Geometry: final body of the model. Coordinates: model frame, mm. A direction names the side the tool comes from. Round coordinates to 2 decimals unless told otherwise and drop trailing zeros. Loops run counter-clockwise (first coordinate to the right, second up) from the corner with the lowest first, then second, coordinate; pieces in that order, holes last. Notation, with made-up numbers: (71, 79) - (105, 79) arc R32 ccw to (105, 112) - close; hole circle Ø5 at (-3, 21.5). An arc over 180 degrees is marked (long way). Use CSV: the item, a comma, the result in double quotes.
from build123d import *

# Parameters (mm, degrees)
F1_DEPTH  = 1.5875
F3_DEPTH  = 4.7625
F4_W      = 6.35
F4_H      = 6.35
F5_DEPTH  = 3.175
F6_SIZE   = 1.8598642
F7_W      = 28.575
F7_H      = 3.175
F8_DEPTH  = 1.5875
F9_W      = 25.4
F9_H      = 1.5875
F10_DEPTH = 7.9375
F11_R     = 1.0922
F11_R_2   = 1.63322
F12_DEPTH = 28.575
F13_SIZE  = 1.58749
F14_R     = 0.396875
F15_DEPTH = 7.9375
F16_R     = 1.63322
F17_DEPTH = 1.5875


# Not quite as in the source:
# - a fillet or chamfer is up to 0.001 mm smaller than in the source, because OpenCascade refuses the exact size


with BuildPart() as f1:
    # F0 (on Top) → F1 (new body)
    with BuildSketch(Plane.XY):
        Polygon((-87.87765, 25.4), (-127, 25.4), (-127, 20.6375), (-48.7553, 20.6375), (-23.3553, -4.7625), (23.3553, -4.7625), (48.7553, 20.6375), (127, 20.6375), (127, 25.4), (87.87765, 25.4), (46.7826079092, 49.1262336135), (-46.7826079092, 49.1262336135), align=None)
        Polygon((-21.3826079092, 0), (-46.7826079092, 25.4), (-78.35265, 25.4), (-45.5064998802, 44.3637336135), (45.5064998802, 44.3637336135), (78.35265, 25.4), (46.7826079092, 25.4), (21.3826079092, 0), align=None, mode=Mode.SUBTRACT)
    extrude(amount=F1_DEPTH)

    # F2 (on face) → F3 (join)
    with BuildSketch(Plane.XY.offset(1.5875)):
        Polygon((-127, 22.225), (-127, 20.6375), (-48.7553, 20.6375), (-23.3553, -4.7625), (23.3553, -4.7625), (48.7553, 20.6375), (127, 20.6375), (127, 22.225), (93.376911314, 22.225), (87.87765, 25.4), (46.7826079092, 49.1262336135), (-46.7826079092, 49.1262336135), (-87.87765, 25.4), (-93.376911314, 22.225), align=None)
        Polygon((90.201911314, 22.225), (48.0977359697, 22.225), (22.6977359697, -3.175), (14.2875, -3.175), (14.2875, -1.5875), (-14.2875, -1.5875), (-14.2875, -3.175), (-22.6977359697, -3.175), (-48.0977359697, 22.225), (-90.201911314, 22.225), (-46.3572385662, 47.5387336135), (-14.2875, 47.5387336135), (-14.2875, 45.9512336135), (14.2875, 45.9512336135), (14.2875, 47.5387336135), (46.3572385662, 47.5387336135), align=None, mode=Mode.SUBTRACT)
    extrude(amount=F3_DEPTH)

    # F4 (on face) → F5 (join, through all)
    with BuildSketch(Plane(origin=(0, 22.225, 0), x_dir=(-1, 0, 0), z_dir=(0, 1, 0))):
        with Locations((-53.5178, 3.175)):
            Rectangle(F4_W, F4_H)
        with Locations((-123.825, 3.175)):
            Rectangle(F4_W, F4_H)
        with Locations((123.825, 3.175)):
            Rectangle(F4_W, F4_H)
        with Locations((53.5178, 3.175)):
            Rectangle(F4_W, F4_H)
    extrude(amount=F5_DEPTH)

    # F6
    f6_edges = [f1.edges().sort_by_distance(p)[0] for p in [
        (-127, 23.01875, 6.35),
        (-120.65, 23.8125, 6.35),
        (-56.6928, 23.8125, 6.35),
        (-50.3428, 23.8125, 6.35),
        (50.3428, 23.8125, 6.35),
        (56.6928, 23.8125, 6.35),
        (120.65, 23.8125, 6.35),
        (127, 23.01875, 6.35),
    ]]
    chamfer(f6_edges, length=F6_SIZE)

    # F7 (on face) → F8 (join)
    with BuildSketch(Plane.XY.offset(6.35)):
        with Locations((0, -3.175)):
            Rectangle(F7_W, F7_H)
        with Locations((0, 47.5387336135)):
            Rectangle(F7_W, F7_H)
    extrude(amount=F8_DEPTH)

    # F9 (on face) → F10 (cut, through all)
    with BuildSketch(Plane.XY.offset(7.9375)):
        with Locations((0, -3.96875)):
            Rectangle(F9_W, F9_H)
        with Locations((0, 48.3324836135)):
            Rectangle(F9_W, F9_H)
    extrude(amount=-F10_DEPTH, mode=Mode.SUBTRACT)

    # F11 (on face) → F12 (cut, through all)
    with BuildSketch(Plane.XZ.offset(3.175)):
        with Locations((53.5178, 3.175)):
            Circle(F11_R)
        with Locations((123.825, 3.175)):
            Circle(F11_R)
        with Locations((-123.825, 3.175)):
            Circle(F11_R)
        with Locations((-53.5178, 3.175)):
            Circle(F11_R)
        with Locations((0, 4.7625)):
            Circle(F11_R_2)
    extrude(amount=-F12_DEPTH, mode=Mode.SUBTRACT)

    # F13 (size 1.5875 in the source; OpenCascade refuses exactly that, so slightly less here)
    f13_edges = [f1.edges().sort_by_distance(p)[0] for p in [
        (-14.2875, -3.96875, 6.35),
        (14.2875, -3.96875, 6.35),
        (-14.2875, 48.332484, 6.35),
        (14.2875, 48.332484, 6.35),
    ]]
    chamfer(f13_edges, length=F13_SIZE)

    # F14 (on face) → F15 (cut, through all)
    with BuildSketch(Plane.XY.offset(7.9375)):
        with Locations((-12.7, -3.175)):
            Circle(F14_R)
        with Locations((12.7, -3.175)):
            Circle(F14_R)
        with Locations((12.7, 47.5387336135)):
            Circle(F14_R)
        with Locations((-12.7, 47.5387336135)):
            Circle(F14_R)
    extrude(amount=-F15_DEPTH, mode=Mode.SUBTRACT)

    # F16 (on face) → F17 (cut, through all)
    with BuildSketch(Plane(origin=(0, 47.5387336135, 0), x_dir=(-1, 0, 0), z_dir=(0, 1, 0))):
        with Locations((0, 4.7625)):
            Circle(F16_R)
    extrude(amount=-F17_DEPTH, mode=Mode.SUBTRACT)


solid = f1.part
Item 1: Section B-B on y = 42. Return the cut outline in (x, z).
Final values:
outline,"(-59.13, 0) - (-49.6, 0) - (-49.6, 1.59) - (-55.95, 1.59) - (-55.95, 6.35) - (-59.13, 6.35) - close; (49.6, 0) - (59.13, 0) - (59.13, 6.35) - (55.95, 6.35) - (55.95, 1.59) - (49.6, 1.59) - close"
Item 2: Material intervals for line 1 (Y direction, x = 15, z = 5.5) (1 decimal); line 2 (Z direction, x = 71, y = 32.5); line 3 (Y direction, x = 71, z = 1), sorted ascending.
Final values:
line 1,"y = -4.8 to -3.2, 47.5 to 49.1"
line 2,"z = 0 to 1.59"
line 3,"y = 20.64 to 25.4, 29.65 to 35.14"
Item 3: Pin query (flat end, axial travel): P1, Ø2, axis at y = 5, z = 7, coming from the -X side; P2, Ø1.6, axis at x = -102, y = 24.5, coming from the +Z side; P3, Ø1.3, axis at x = 0, z = 1, coming from the +Y side. Return the tip coordinate at first contact, or that it passes through.
Final values:
P1,"stops at x = -33.88"
P2,"stops at z = 1.59"
P3,"stops at y = 47.54"
Item 4: Section A-A on x = 6.5. Return the cut outline in (y, z) (1 decimal).
Final values:
outline,"(-3.2, 0) - (0, 0) - (0, 1.6) - (-1.6, 1.6) - (-1.6, 7.9) - (-3.2, 7.9) - close; (44.4, 0) - (47.5, 0) - (47.5, 7.9) - (46, 7.9) - (46, 1.6) - (44.4, 1.6) - close"
Item 5: Mould query, pull axis X, two halves, no side actions, for faces 5 (the flat face through (30, 47.539, 4)), 6 (the flat face through (18, -4.762, 3)). Classes: released by +X, released by -X, zero draft, split by the parting line, or undercut.
Final values:
face 5,"undercut"
face 6,"zero draft"
Item 6: Reachability of faces 1 (the flat face through (-31, 47.539, 4)), 2 (the flat face through (61.7, 35.015, 0.783)), 3 (the flat face through (-108, 22.225, 4)), 4 (the flat face through (-88, 20.638, 3)) from +Z, -Z, +X, -X, +Y, -Y: full face, straight path, thin tool, end or side. Return the list, or none.
Final values:
face 1,"+Z"
face 2,"+Z, -Z"
face 3,"+Z, +Y"
face 4,"+Z, -Z, -X, -Y"
